Autodesk Inventor part; units mm, degrees
ref_plane "YZ Plane" through (0, 0, 0) normal (1, 0, 0) x (0, 1, 0)
ref_plane "XZ Plane" through (0, 0, 0) normal (0, 1, 0) x (-1, 0, 0)
ref_plane "XY Plane" through (0, 0, 0) normal (0, 0, 1) x (1, 0, 0)
sketch "Sketch1" plane through (0, 0, 0) normal (0, 0, 1) x (1, 0, 0)
  line L0 (0, 0) -> (82.55, 0)
  line L1 (82.55, 0) -> (82.55, 57.15)
  line L2 (82.55, 57.15) -> (0, 57.15)
  line L3 (0, 57.15) -> (0, 0)
  dimension "d0" = 57.15
  dimension "d1" = 82.55
extrude "Extrusion1" add sketch "Sketch1" along normal blind 9.525
sketch "Sketch2" plane through (0, 0, 9.525) normal (0, 0, 1) x (1, 0, 0)
  line L0 (-21.536, 28.575) -> (122.8285, 28.575) construction
  line L1 (82.55, 57.15) -> (0, 57.15) construction
  line L2 (0, 57.15) -> (0, 0)
  line L3 (82.55, 0) -> (82.55, 57.15)
  line L4 (0, 26.9875) -> (82.55, 26.9875)
  line L5 (82.55, 26.9875) -> (82.55, 30.1625)
  line L6 (82.55, 30.1625) -> (0, 30.1625)
  line L7 (0, 30.1625) -> (0, 26.9875)
  dimension "d4" = 28.575
  dimension "d5" = 1.5875
  dimension "d6" = 1.5875
extrude "Extrusion2" cut sketch "Sketch2" against normal blind 3.175
properties part number "000106"
Source: CAD feature listing. Evaluate the final solid. Frame: model axes, mm. A direction names the side the tool comes from. Round coordinates to 2 decimals unless told otherwise and drop trailing zeros. Order: outer loops, then holes, each group sorted by start corner. A loop starts at its lowest first (then second) coordinate and runs counter-clockwise, first axis right, second up. Notation, with made-up numbers: (31.5, 37) -> (67.5, 37) arc R20 cw to (67.5, 45) -> close; hole circle Ø6 at (65.25, -20). An arc over 180 degrees is marked (long way). One line per item, written item: value. Start each with the question number.
Q1. Access query for faces 4 (the flat face through (41, 0, 5)), 5 (the flat face through (41, 29, 6.35)). Directions: +Z, -Z, +X, -X, +Y, -Y. A direction counts if a zero-diameter tool reaches every point of the face in a straight line with its end or side. Return the directions, or none.
Q2. Pin query (flat end, axial travel): pin 1 (1 mm diameter, centred on x = 37.5, y = 28, fed in from +Z). Return the tip coordinate at first contact, or that it passes through.
Q3. Draft query along Z for faces 1 (the flat face through (41, 26.988, 8)), 2 (the flat face through (41, 29, 0)), 3 (the flat face through (41, 14, 9.525)). Return one class per face: pulls with the +Z half, pulls with the -Z half, needs draft (parallel to the pull), parting line crosses it, or undercut.
Q4. Section query A-A (z = 8.25). Return the cut outline in (x, y), plus the area to 3 significant figures.
Q5. Material intervals for probe 1 along Z at (x, y) = (51, 28), sorted ascending.
Findings below:
1. face 4: +Z, -Z, +X, -X, -Y
1. face 5: +Z, +X, -X
2. pin 1: z = 6.35
3. face 1: needs draft
3. face 2: pulls with the -Z half
3. face 3: pulls with the +Z half
4. outline: (0, 0) -> (82.55, 0) -> (82.55, 26.99) -> (0, 26.99) -> close; (0, 30.16) -> (82.55, 30.16) -> (82.55, 57.15) -> (0, 57.15) -> close
4. area: 4,460 mm²
5. probe 1: 0 to 6.35
